Verification items for the finished model (mm, model axes). Face numbers are marked on the shaded views. A direction names the side the tool comes from. Coordinates: 2 decimals unless noted, no trailing zeros. Order: outer loops, then holes, each group sorted by start corner. A loop starts at its lowest first (then second) coordinate and runs counter-clockwise, first axis right, second up. Notation, with made-up numbers: (13.5, 42.5) -> (54.5, 42.5) arc R4 cw to (54.5, 46.5) -> close; hole circle Ø6 at (-32, -11.75). An arc over 180 degrees is marked (long way). Use CSV: the item, a comma, the result in double quotes. Start each with the question number.
1) Sectioned sample at B-B on z = -7.77. Record the boundary of the cut face in (x, y), then the cut area to 3 significant figures.
2) Sectioned sample at C-C on y = 18.95. Record the boundary of the cut face in (x, z), then the cut area to 3 significant figures.
3) Release check for a two-part mould opening along Z. For the marked faces 1, 2, 3 and 4 record: released by +Z, released by -Z, zero draft, split by the parting line, or undercut.
4) Scan lines: line 1 along Y through (x, z) = (9, -7.77); line 2 along Z through (x, y) = (7.5, 28.5); line 3 along Z through (x, y) = (8.5, 17.5). Record each from-to range of solid material in increasing order.
5) Go/stop test with flat-tipped pins: pin 1 (2 mm diameter, centred on x = 12, z = -12, fed in from -Y); pin 2 (4 mm diameter, centred on x = 7.5, y = 16, fed in from -Z); pin 3 (1.9 mm diameter, centred on x = 9.5, y = 1.5, fed in from -Z); pin 4 (1 mm diameter, centred on x = 11.5, y = 16.5, fed in from -Z). Record where each tip stops, or that it passes through.
6) Sectioned sample at A-A on x = 7.25. Record the boundary of the cut face in (y, z).
7) Tool access check on the marked faces 5 and 6. Record the directions out of +Z, -Z, +X, -X, +Y, -Y that give a thin tool (end or side, any length) a straight path to the whole face; none if there is none.
from build123d import *

# Parameters (mm, degrees)
SKETCH1_W           = 17.78
SKETCH1_H           = 15.54
BOSS_EXTRUDE1_DEPTH = 3.1
SKETCH3_R           = 13.85
BOSS_EXTRUDE2_DEPTH = 17.78
FILLET1_R           = 2.54


with BuildPart() as part:
    # Sketch1 → Boss-Extrude1 (new body)
    with BuildSketch(Plane(origin=(0, 0, 0), x_dir=(1, 0, 0), z_dir=(0, 1, 0))):
        with Locations((8.89, 7.77)):
            Rectangle(SKETCH1_W, SKETCH1_H)
    extrude(amount=BOSS_EXTRUDE1_DEPTH)

    # Sketch3 → Boss-Extrude2 (add)
    with BuildSketch(Plane.ZY):
        with BuildLine():
            Line((-15.54, 3.1), (-15.54, 5.135167392))
            ThreePointArc((-15.54, 5.135167392), (-7.77, 34.8), (0, 5.135167392))
            Line((0, 5.135167392), (0, 3.1))
            Line((0, 3.1), (-15.54, 3.1))
        make_face()
        with Locations((-7.77, 18.95)):
            Circle(SKETCH3_R, mode=Mode.SUBTRACT)
    extrude(amount=-BOSS_EXTRUDE2_DEPTH)

    # Fillet1
    fillet1_edges = [part.edges().sort_by_distance(p)[0] for p in [
        (8.89, 5.135167392, 0),
        (8.89, 5.135167392, -15.54),
    ]]
    fillet(fillet1_edges, radius=FILLET1_R)


solid = part.part
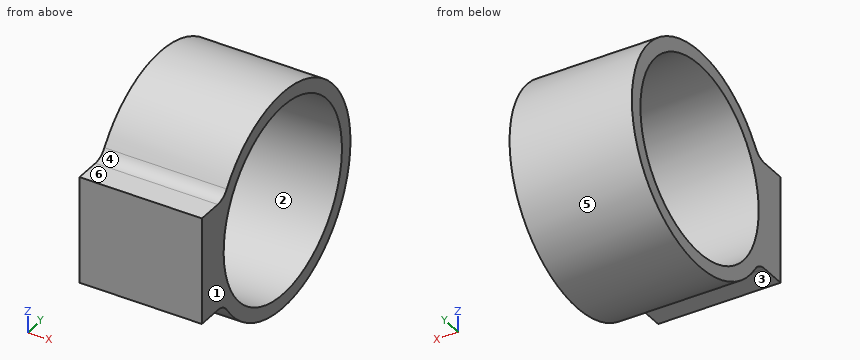
Answers follow:
1,outline,"(0, 0) -> (17.78, 0) -> (17.78, 5.1) -> (0, 5.1) -> close; (0, 32.8) -> (17.78, 32.8) -> (17.78, 34.8) -> (0, 34.8) -> close"
1,area,"126 mm²"
2,outline,"(0, -23.62) -> (17.78, -23.62) -> (17.78, -21.62) -> (0, -21.62) -> close; (0, 6.08) -> (17.78, 6.08) -> (17.78, 8.08) -> (0, 8.08) -> close"
2,area,"71.1 mm²"
3,face 1,"zero draft"
3,face 2,"undercut"
3,face 3,"released by -Z"
3,face 4,"released by +Z"
4,line 1,"y = 0 to 5.1, 32.8 to 34.8"
4,line 2,"z = -20.42 to -17.8, 2.26 to 4.88"
4,line 3,"z = -23.55 to -21.54, 6 to 8.01"
5,pin 1,"stops at y = 0"
5,pin 2,"stops at z = -23.59"
5,pin 3,"stops at z = -15.54"
5,pin 4,"stops at z = -23.5"
6,outline,"(0, -15.54) -> (3.72, -15.54) arc R2.54 cw to (5.83, -16.66) arc R15.85 ccw (long way) to (5.83, 1.12) arc R2.54 cw to (3.72, 0) -> (0, 0) -> close; hole circle Ø27.7 at (18.95, -7.77)"
7,face 5,"+X, -X"
7,face 6,"+Z, +X, -X, -Y"
